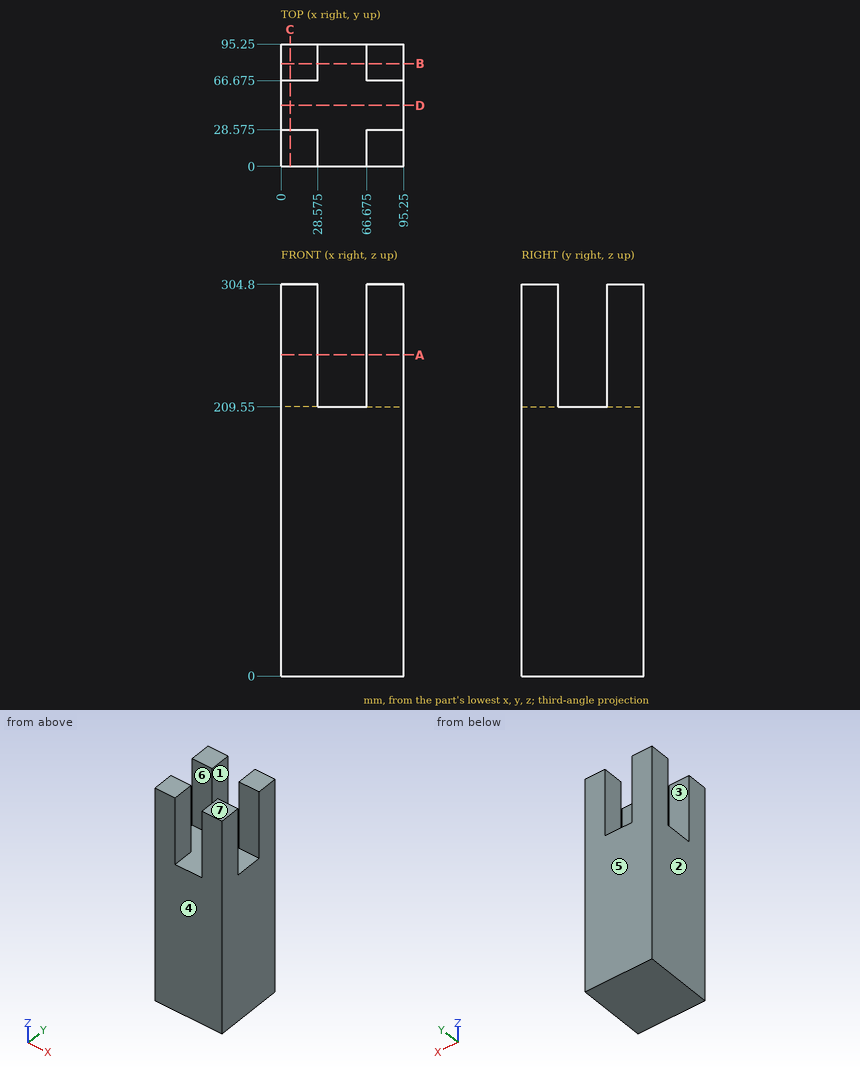
Source: three-view drawing plus pictorial views. Frame: mm from the lowest corner of the part. A direction names the side the tool comes from. Coordinates: 2 decimals unless noted, no trailing zeros. Write each loop counter-clockwise with the first axis right and the second up, starting at its lowest first coordinate (ties: lowest second). Pieces come first, ordered by that corner, then holes. Notation, with made-up numbers: (67, 56.5) - (119, 56.5) arc R28 cw to (119, 91.5) - close; hole circle Ø5 at (7, 27). An arc over 180 degrees is marked (long way). Return JSON: item names as keys, results as strings.
Item 1: Section query D-D (y = 47.5). Output: boundary loops of the cut face in (x, z), and give its area (3 significant figures).
Completed:
{"outline": "(0, 0) - (95.25, 0) - (95.25, 209.55) - (0, 209.55) - close", "area": "20,000 mm2"}
Item 2: Reachability of the marked faces 1, 2 and 3 from +Z, -Z, +X, -X, +Y, -Y: full face, straight path, thin tool, end or side. Return the list, or none.
Completed:
{"face 1": "+Z, +Y, -Y", "face 2": "+Z, -Z, -X, +Y, -Y", "face 3": "+Z, +X, -X"}
Item 3: Pin query (flat end, axial travel): pin 1 Ø4 at (x, y) = (62.5, 72) entering from +Z. Return the tip coordinate at first contact, or that it passes through.
Completed:
{"pin 1": "stops at z = 209.55"}
Item 4: Line query: L1, parallel to Y at x = 10.5, z = 285 (3 decimals); L2, parallel to Z at x = 51.5, y = 84. Output: solid intervals per line, ascending.
Completed:
{"L1": "y = 0 to 28.575, 66.675 to 95.25", "L2": "z = 0 to 209.55"}
Item 5: Pull-direction query (Y, two-part tool) for the marked faces 4, 5, 6 and 7; classes: +Y half, -Y half, draft (parallel to the pull), parting line (faces both ways), or undercut.
Completed:
{"face 4": "-Y half", "face 5": "+Y half", "face 6": "undercut", "face 7": "draft"}
Item 6: Section query B-B (y = 80). Output: boundary loops of the cut face in (x, z) (3 decimals).
Completed:
{"outline": "(0, 0) - (95.25, 0) - (95.25, 304.8) - (66.675, 304.8) - (66.675, 209.55) - (28.575, 209.55) - (28.575, 304.8) - (0, 304.8) - close"}
Item 7: Section query A-A (z = 250). Output: boundary loops of the cut face in (x, y) (3 decimals), and give its area (3 significant figures).
Completed:
{"outline": "(0, 0) - (28.575, 0) - (28.575, 28.575) - (0, 28.575) - close; (0, 66.675) - (28.575, 66.675) - (28.575, 95.25) - (0, 95.25) - close; (66.675, 0) - (95.25, 0) - (95.25, 28.575) - (66.675, 28.575) - close; (66.675, 66.675) - (95.25, 66.675) - (95.25, 95.25) - (66.675, 95.25) - close", "area": "3,270 mm2"}
